```python
from build123d import *

# Parameters (mm, degrees)
F0_R     = 50.8
F1_DEPTH = 127
F2_DEPTH = 101.6
F3_DEPTH = 152.4
F4_DEPTH = 25.4


with BuildPart() as f1:
    # F0 (on Front) → F1 (new body)
    with BuildSketch(Plane.XZ):
        with BuildLine():
            ThreePointArc((-42.247934, -96.137584), (5.377066, -70.936803), (24.427066, -20.53524))
            ThreePointArc((24.427066, -20.53524), (24.267038, -15.599377), (23.787624, -10.684245))
            ThreePointArc((23.787624, -10.684245), (-51.772934, 55.66476), (-127.333492, -10.684245))
            ThreePointArc((-127.333492, -10.684245), (-112.067679, -67.129056), (-61.297934, -96.137584))
            ThreePointArc((-61.297934, -96.137584), (-51.772934, -96.73524), (-42.247934, -96.137584))
        make_face()
        with Locations((-51.772934, -20.53524)):
            Circle(F0_R, mode=Mode.SUBTRACT)
    extrude(amount=F1_DEPTH)

    # F0 (on Front) → F2 (join)
    with BuildSketch(Plane.XZ):
        with BuildLine():
            Line((-42.247934, -223.73524), (-42.247934, -96.137584))
            ThreePointArc((-42.247934, -96.137584), (-51.772934, -96.73524), (-61.297934, -96.137584))
            Line((-61.297934, -96.137584), (-61.297934, -223.73524))
            Line((-61.297934, -223.73524), (-42.247934, -223.73524))
        make_face()
    extrude(amount=F2_DEPTH)

    # F0 (on Front) → F3 (join)
    with BuildSketch(Plane.XZ):
        Polygon((97.452066, -274.53524), (97.452066, -223.73524), (-42.247934, -223.73524), (-61.297934, -223.73524), (-200.997934, -223.73524), (-200.997934, -274.53524), align=None)
    extrude(amount=F3_DEPTH)

    # F0 (on Front) → F4 (join)
    with BuildSketch(Plane.XZ):
        with BuildLine():
            ThreePointArc((-61.297934, -96.137584), (-112.067679, -67.129056), (-127.333492, -10.684245))
            Line((-127.333492, -10.684245), (-200.997934, -223.73524))
            Line((-200.997934, -223.73524), (-61.297934, -223.73524))
            Line((-61.297934, -223.73524), (-61.297934, -96.137584))
        make_face()
        with BuildLine():
            ThreePointArc((23.787624, -10.684245), (24.267038, -15.599377), (24.427066, -20.53524))
            ThreePointArc((24.427066, -20.53524), (5.377066, -70.936803), (-42.247934, -96.137584))
            Line((-42.247934, -96.137584), (-42.247934, -223.73524))
            Line((-42.247934, -223.73524), (97.452066, -223.73524))
            Line((97.452066, -223.73524), (23.787624, -10.684245))
        make_face()
    extrude(amount=F4_DEPTH)


solid = f1.part
```
The listing builds one solid part. Answer for the finished solid, in the listing's coordinates (mm). A direction names the side the tool comes from. Coordinates: 2 decimals unless noted, no trailing zeros. Write each loop counter-clockwise with the first axis right and the second up, starting at its lowest first coordinate (ties: lowest second). Pieces come first, ordered by that corner, then holes. Notation, with made-up numbers: (-35, 79.25) - (-27, 79.25) arc R8 ccw to (-27, 92.25) - close; hole circle Ø10 at (25, 78.25). An arc over 180 degrees is marked (long way). Return JSON: item names as keys, results as strings. Group by question number.
Q1. The part is cut by section C-C on z = -57. Write down the section's boundary in (x, y).
Q2. The part is cut by section D-D on y = -39. Write down the section's boundary in (x, z).
Q3. For a pull along Z with two mould halves and no side action, classify faces 6 (the flat face through (97.452, -75, -249)), 7 (the flat face through (-163.65, -12.52, -115.72)), 8 (the flat face through (-61.298, -63, -159)) as +Z half, -Z half, draft (parallel to the pull), parting line (faces both ways), or undercut.
Q4. The part is cut by section A-A on y = -122. Write down the section's boundary in (x, z).
Q5. Flat-ended cylindrical pins translate along their axes: pin 1 Ø15 at (x, z) = (-47.5, -151.5) entering from -Y; pin 2 Ø12 at (y, z) = (-111.5, -36.5) entering from +X; pin 3 Ø5 at (y, z) = (-51.5, -193.5) entering from -X. Find the tip coordinate at first contact, or state that the pin passes through.
Q6. Which of the six approach directions +Z, -Z, +X, -X, +Y, -Y give full straight-line access (tool end or side, diameter ignored) to faces 1 (the cylindrical face through (-51.907, -114.122, -96.735)), 2 (the flat face through (-52, -101.6, -159)), 3 (the cylindrical face through (24.27, -75.49, -15.67)), 4 (the flat face through (-36, -127, -70)), 5 (the cylindrical face through (4.864, -75.489, -71.512))?
Q7. Find the intervals of material crossed by line 1 along Z through (x, y) = (-86.5, -74); line 2 along Z through (x, y) = (-17, -122); line 3 along X through (y, z) = (-29, -222.5), in increasing order. Write a range as [from, to].
Q8. The part is cut by section B-B on x = -14. Write down the section's boundary in (y, z).
Evaluation:
{
 "1": {"outline": "(-143.35, -25.4) - (-118.68, -25.4) - (-118.68, -127) - (-87.14, -127) - (-87.14, 0) - (-143.35, 0) - close; (-16.4, -127) - (15.14, -127) - (15.14, -25.4) - (39.8, -25.4) - (39.8, 0) - (-16.4, 0) - close"},
 "2": {"outline": "(-201, -274.54) - (97.45, -274.54) - (97.45, -223.74) - (-42.25, -223.74) - (-42.25, -96.14) arc R76.2 ccw to (24.43, -20.54) arc R76.2 ccw to (23.79, -10.68) arc R76.2 ccw to (-127.33, -10.68) arc R76.2 ccw to (-61.3, -96.14) - (-61.3, -223.74) - (-201, -223.74) - close; hole circle Ø101.6 at (-51.77, -20.54)"},
 "3": {"face 6": "draft", "face 7": "+Z half", "face 8": "undercut"},
 "4": {"outline": "(-201, -274.54) - (97.45, -274.54) - (97.45, -223.74) - (-201, -223.74) - close; (-127.33, -10.68) arc R76.2 ccw to (-61.3, -96.14) arc R76.2 ccw to (-42.25, -96.14) arc R76.2 ccw to (24.43, -20.54) arc R76.2 ccw to (23.79, -10.68) arc R76.2 ccw to start; hole circle Ø101.6 at (-51.77, -20.54)"},
 "5": {"pin 1": "stops at y = -101.6", "pin 2": "stops at x = 23.77", "pin 3": "stops at x = -61.3"},
 "6": {"face 1": "-Y", "face 2": "+X, -X, -Y", "face 3": "+Z, +X, -Y", "face 4": "+Z, +X, -X, -Y", "face 5": "+X, -Y"},
 "7": {"line 1": "z = [-274.54, -223.74], [-88.36, -57.61], [16.54, 47.29]", "line 2": "z = [-274.54, -223.74], [-88.34, -57.57], [16.5, 47.27]", "line 3": "x = [-61.3, -42.25]"},
 "8": {"outline": "(-152.4, -274.54) - (0, -274.54) - (0, -54.5) - (-127, -54.5) - (-127, -86.71) - (-25.4, -86.71) - (-25.4, -223.74) - (-152.4, -223.74) - close; (-127, 13.43) - (0, 13.43) - (0, 45.64) - (-127, 45.64) - close"}
}
